from build123d import *

# Parameters (mm, degrees)
SKETCH_W        = 103
SKETCH_H        = 30.3
PAD_DEPTH       = 1.62
SKETCH001_R     = 2.1
POCKET_DEPTH    = 5
SKETCH002_R     = 1.45
SKETCH002_W     = 18.34
SKETCH002_H     = 11.81
SKETCH002_W_2   = 10.5
SKETCH002_H_2   = 9.5
POCKET001_DEPTH = 5
FILLET_R        = 4


with BuildPart() as part:
    # Sketch → Pad (new body)
    with BuildSketch(Plane.XY):
        Rectangle(SKETCH_W, SKETCH_H)
    extrude(amount=PAD_DEPTH)

    # Sketch001 → Pocket (cut)
    with BuildSketch(Plane.XY.offset(1.62)):
        with Locations((-47.51, 11.26)):
            Circle(SKETCH001_R)
        with Locations((47.51, 11.26)):
            Circle(SKETCH001_R)
        with Locations((-47.51, -11.26)):
            Circle(SKETCH001_R)
        with Locations((47.51, -11.26)):
            Circle(SKETCH001_R)
    extrude(amount=-POCKET_DEPTH, mode=Mode.SUBTRACT)

    # Sketch002 → Pocket001 (cut)
    with BuildSketch(Plane.XY.offset(1.62)):
        with Locations((-5.364, -2.35)):
            Circle(SKETCH002_R)
        with Locations((0.478, -2.35)):
            Circle(SKETCH002_R)
        with Locations((14.448, -2.35)):
            Circle(SKETCH002_R)
        with Locations((-24.003, 2.805)):
            Rectangle(SKETCH002_W, SKETCH002_H)
        with Locations((27.94, 1.65)):
            Rectangle(SKETCH002_W_2, SKETCH002_H_2)
    extrude(amount=-POCKET001_DEPTH, mode=Mode.SUBTRACT)

    # Fillet
    fillet_edges = [part.edges().sort_by_distance(p)[0] for p in [
        (-51.5, -15.15, 0.81),
        (-51.5, 15.15, 0.81),
        (51.5, -15.15, 0.81),
        (51.5, 15.15, 0.81),
    ]]
    fillet(fillet_edges, radius=FILLET_R)


solid = part.part
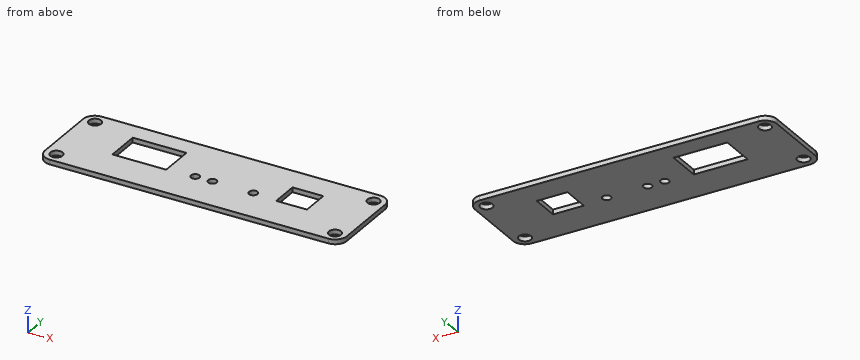
Here's how the part is built. I have some questions about the finished solid (model axes, mm). Round coordinates to 2 decimals unless told otherwise and drop trailing zeros. Write each loop counter-clockwise with the first axis right and the second up, starting at its lowest first coordinate (ties: lowest second). Pieces come first, ordered by that corner, then holes.
1. Suppose I cut it at C-C (z = 0.8). State how many separate pieces and enclosed holes the cut face has, and give its area (3 significant figures).
2. I need wall thicknesses on L1, parallel to X at y = 2, z = 0.5; L2, parallel to Y at x = 47.51, z = 0.95; L3, parallel to X at y = -12.5, z = 1.45. Which ranges of each line are inside material? Lowest first, please.
3. Suppose I cut it at B-B (x = -17.5). List the corners of the cut face in (y, z) for me, and give its area (3 significant figures).
4. Suppose I cut it at D-D (y = -12.5). List the corners of the cut face in (x, z) for me, and give its area (3 significant figures).
5. Suppose I cut it at A-A (y = 7.5). List the corners of the cut face in (x, z) for me, and give its area (3 significant figures).
Answer sheet:
1. separate pieces: 1
1. enclosed holes: 9
1. area: 2,720 mm2
2. L1: x = -51.5 to -33.17, -14.83 to 22.69, 33.19 to 51.5
2. L2: y = -15.15 to -13.36, -9.16 to 9.16, 13.36 to 15.15
2. L3: x = -51.27 to -49.2, -45.82 to 45.82, 49.2 to 51.27
3. outline: (-15.15, 0) - (-3.1, 0) - (-3.1, 1.62) - (-15.15, 1.62) - close; (8.71, 0) - (15.15, 0) - (15.15, 1.62) - (8.71, 1.62) - close
3. area: 30.0 mm2
4. outline: (-51.27, 0) - (-49.2, 0) - (-49.2, 1.62) - (-51.27, 1.62) - close; (-45.82, 0) - (45.82, 0) - (45.82, 1.62) - (-45.82, 1.62) - close; (49.2, 0) - (51.27, 0) - (51.27, 1.62) - (49.2, 1.62) - close
4. area: 155 mm2
5. outline: (-51.5, 0) - (-33.17, 0) - (-33.17, 1.62) - (-51.5, 1.62) - close; (-14.83, 0) - (51.5, 0) - (51.5, 1.62) - (-14.83, 1.62) - close
5. area: 137 mm2
